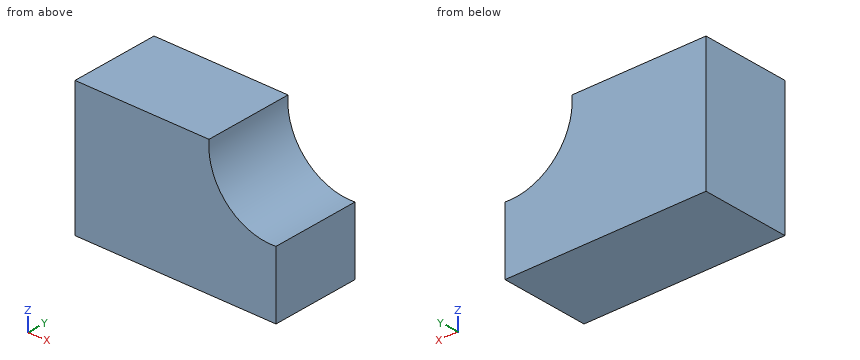
```python
from build123d import *

# Parameters (mm, degrees)
F0_W     = 57.15
F0_H     = 38.1
F1_DEPTH = 25.4
F3_DEPTH = 25.4
F4_W     = 15.0772607885
F4_H     = 19.0978627652
F5_DEPTH = 107
F7_DEPTH = 107
F8_W     = 12.6649001613
F8_H     = 19.2988961935
F9_DEPTH = 107


# Not quite as in the source:
# - an extrude ends at something that could not be found from the text; its depth is read off the source's solid


with BuildPart() as f1:
    # F0 (on Front) → F1 (new body)
    with BuildSketch(Plane.XZ):
        with Locations((28.575, 19.05)):
            Rectangle(F0_W, F0_H)
    extrude(amount=F1_DEPTH)

    # F2 (on face) → F3 (cut)
    with BuildSketch(Plane.XZ.offset(25.4)):
        with BuildLine():
            Line((57.15, 38.1), (38.1, 38.1))
            ThreePointArc((38.1, 38.1), (43.2045261365, 24.1545261365), (57.15, 19.05))
            Line((57.15, 19.05), (57.15, 38.1))
        make_face()
    extrude(amount=-F3_DEPTH, mode=Mode.SUBTRACT)

    # F4 (on Right) → F5 (cut, through all)
    with BuildSketch(Plane.YZ):
        with Locations((-12.0618094224, 28.9483414963)):
            Rectangle(F4_W, F4_H)
    extrude(amount=-F5_DEPTH, mode=Mode.SUBTRACT)

    # F6 (on Right) → F7 (cut, through all)
    with BuildSketch(Plane.YZ):
        Polygon((-6.7345094867, 37.8941856325), (-18.3942597359, 38.2962450385), (-18.3942597359, 24.6261935681), (-6.7345094867, 24.6261935681), align=None)
    extrude(amount=-F7_DEPTH, mode=Mode.SUBTRACT)

    # F8 (on Right) → F9 (cut, through all)
    with BuildSketch(Plane.YZ):
        with Locations((-11.2576889805, 28.6467969418)):
            Rectangle(F8_W, F8_H)
    extrude(amount=-F9_DEPTH, mode=Mode.SUBTRACT)


solid = f1.part
```
Geometry: final body of the model. Coordinates: model frame, mm. Coordinates: 2 decimals unless noted, no trailing zeros. Order: outer loops, then holes, each group sorted by start corner. A loop starts at its lowest first (then second) coordinate and runs counter-clockwise, first axis right, second up. Notation, with made-up numbers: M 32.25,17 L 89.25,17 A7 ccw 89.25,22 Z; hole C 11.25,-4.5 d1. An arc over 180 degrees is marked long. Answer in a Markdown table with one row per item. Add a question column.
Q1. Contact query for flat-ended pins moving along their axis: P1, Ø8, axis at x = 51.5, y = -5.5, coming from the +Z side; P2, Ø1.5, axis at x = 40, z = 33.5, coming from the -Y side. Output: stop coordinate, or through.
Q2. Section query A-A on y = -5. Return the cut outline in (x, z), and give its area (3 significant figures).
Q3. Section query B-B on x = 53. Return the cut outline in (y, z).
Q4. Section query C-C on z = 36.5. Return the cut outline in (x, y), and give its area (3 significant figures).
Q5. Line query: L1, parallel to Z at x = 55, y = -22.25; L2, parallel to Z at x = 44.5, y = -7; L3, parallel to X at y = -9, z = 26.5. Output: solid intervals per line, ascending.
Completed:
| question | item | result |
|---|---|---|
| 1 | P1 | stops at z = 21 |
| 1 | P2 | passes through |
| 2 | outline | M 0,0 L 57.15,0 L 57.15,19.05 A17.64 cw 38.1,38.1 L 0,38.1 Z |
| 2 | area | 1,880 mm2 |
| 3 | outline | M -25.4,0 L 0,0 L 0,19.19 L -25.4,19.19 Z |
| 4 | outline | M 0,-25.4 L 38.04,-25.4 L 38.04,0 L 0,0 Z |
| 4 | area | 966 mm2 |
| 5 | L1 | z = 0 to 19 |
| 5 | L2 | z = 0 to 22.98 |
| 5 | L3 | x = 0 to 41.24 |
